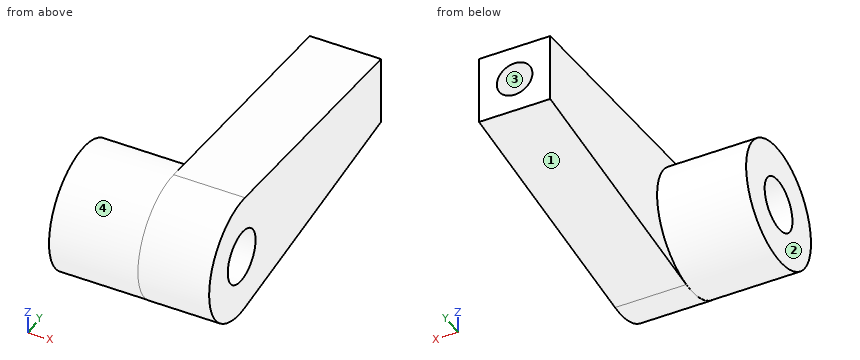
```python
from build123d import *

# Parameters (mm, degrees)
SKETCH1_R           = 3
BOSS_EXTRUDE1_DEPTH = 8
SKETCH2_R           = 7
SKETCH2_R_2         = 3
BOSS_EXTRUDE2_DEPTH = 10
SKETCH3_R           = 2
CUT_EXTRUDE1_DEPTH  = 22


with BuildPart() as part:
    # Sketch1 → Boss-Extrude1 (new body)
    with BuildSketch(Plane(origin=(0, 0, 0), x_dir=(0, 0, -1), z_dir=(1, 0, 0))):
        with BuildLine():
            Line((-4, 0), (-6.981160767, -29.34898091))
            ThreePointArc((-6.981160767, -29.34898091), (0, -37.075184621), (6.981160767, -29.34898091))
            Line((6.981160767, -29.34898091), (4, 0))
            Line((4, 0), (-4, 0))
        make_face()
        with Locations((0, -30.058101362)):
            Circle(SKETCH1_R, mode=Mode.SUBTRACT)
    extrude(amount=-BOSS_EXTRUDE1_DEPTH)

    # Sketch2 → Boss-Extrude2 (add)
    with BuildSketch(Plane.ZY.offset(8)):
        with Locations((0, -30.058101362)):
            Circle(SKETCH2_R)
        with Locations(Location((0, -30.058101362, 0), (0, 0, 180))):
            Circle(SKETCH2_R_2, mode=Mode.SUBTRACT)
    extrude(amount=BOSS_EXTRUDE2_DEPTH)

    # Sketch3 → Cut-Extrude1 (cut)
    with BuildSketch(Plane(origin=(0, 0, 0), x_dir=(1, 0, 0), z_dir=(0, 1, 0))):
        with Locations(Location((-4, 0, 0), (0, 0, 270))):
            Circle(SKETCH3_R)
    extrude(amount=-CUT_EXTRUDE1_DEPTH, mode=Mode.SUBTRACT)


solid = part.part
```
Check sheet for the modelled part. Datum: model origin and axes. Units: mm. Face numbers are marked on the shaded views. Round coordinates to 2 decimals unless told otherwise and drop trailing zeros. Write each loop counter-clockwise with the first axis right and the second up, starting at its lowest first coordinate (ties: lowest second). Pieces come first, ordered by that corner, then holes. Notation, with made-up numbers: (72.25, -36) -> (112.25, -36) arc R23 ccw to (112.25, -25) -> close; hole circle Ø8 at (71, 59.5). An arc over 180 degrees is marked (long way). One line per question, with ' | ' between items. Start each with the question number.
1. Depth check by flat-ended pin: pin 1 (2.5 mm diameter, centred on x = -4, z = 0, fed in from +Y); pin 2 (3 mm diameter, centred on x = -10.5, y = -12.5, fed in from -Z); pin 3 (5 mm diameter, centred on x = -2, y = -18.5, fed in from -Z); pin 4 (3 mm diameter, centred on y = -9.5, z = 5, fed in from -X). Enter the tip coordinate at first touch or a pass-through.
2. Sectioned sample at C-C, the plane x = -2.5. Record the cut outline in (y, z), then the cut area to 3 significant figures.
3. Sectioned sample at D-D, the plane y = -18. Record the cut outline in (x, z).
4. Scan lines: line 1 along Y through (x, z) = (-10, 0); line 2 along Z through (x, y) = (-3.75, -29); line 3 along Z through (x, y) = (-3.5, -3). Record each from-to range of solid material in increasing order. Write a range as from..to.
5. Sectioned sample at B-B, the plane y = -28. Record the cut outline in (x, z), then the cut area to 3 significant figures.
6. Release check for a two-part mould opening along Z. For the marked faces 1, 2, 3 and 4 record: +Z half, -Z half, draft (parallel to the pull), parting line (faces both ways), or undercut.
Taken from the geometry:
1) pin 1: stops at y = -22 | pin 2: passes through | pin 3: stops at z = -6.13 | pin 4: stops at x = -8
2) outline: (-29.35, -6.98) -> (0, -4) -> (0, -1.32) -> (-22, -1.32) -> (-22, 1.32) -> (0, 1.32) -> (0, 4) -> (-29.35, 6.98) arc R7.02 ccw (long way) to start; hole circle Ø6 at (-30.06, 0) | area: 323 mm^2
3) outline: (-8, -5.83) -> (0, -5.83) -> (0, 5.83) -> (-8, 5.83) -> close; hole circle Ø4 at (-4, 0)
4) line 1: y = -37.06..-33.06, -27.06..-23.06 | line 2: z = -6.95..-2.81, 2.81..6.95 | line 3: z = -4.3..-1.94, 1.94..4.3
5) outline: (-18, -6.69) -> (-8, -6.69) -> (-8, -6.84) -> (0, -6.84) -> (0, -2.18) -> (-18, -2.18) -> close; (-18, 2.18) -> (0, 2.18) -> (0, 6.84) -> (-8, 6.84) -> (-8, 6.69) -> (-18, 6.69) -> close | area: 165 mm^2
6) face 1: -Z half | face 2: draft | face 3: undercut | face 4: parting line
